Job drawing, mm, ordinate dimensions from the low corner. One solid piece. A direction names the side the tool comes from. Round coordinates to 2 decimals unless told otherwise and drop trailing zeros. Loops run counter-clockwise (first coordinate to the right, second up) from the corner with the lowest first, then second, coordinate; pieces in that order, holes last.
1) Probe line 1 (Z direction, x = 44.41, y = 1); line 2 (X direction, y = 2.95, z = 3.75); line 3 (Z direction, x = 17.5, y = 3.05). List the from-to ranges inside material, lowest first.
2) Band-saw the part on D-D, the plane x = 17.5. Write the cut outline in (y, z).
3) Band-saw the part on A-A, the plane z = 4. Write the cut outline in (x, y), then the cut area to 3 significant figures.
4) Drop flat-ended pins along their axis: P1, Ø1.5, axis at y = 3.5, z = 3, coming from the +X side; P2, Ø3, axis at x = 44.41, z = 4, coming from the +Y side. Give the stop position or say it passes through.
5) Band-saw the part on B-B, the plane x = 4. Write the cut outline in (y, z), then the cut area to 3 significant figures.
6) 3-axis set-ups, long thin cutter, end or side, ignore diameter. For the marked faces 1, 2 and 3: which of +Z, -Z, +X, -X, +Y, -Y reach the whole face in a straight line?
7) Mould opens along X. For the marked faces 4, 5 and 6 say: +X half, -X half, draft (parallel to the pull), parting line (faces both ways), or undercut.
8) Band-saw the part on C-C, the plane y = 1.65. Write the cut outline in (x, z).
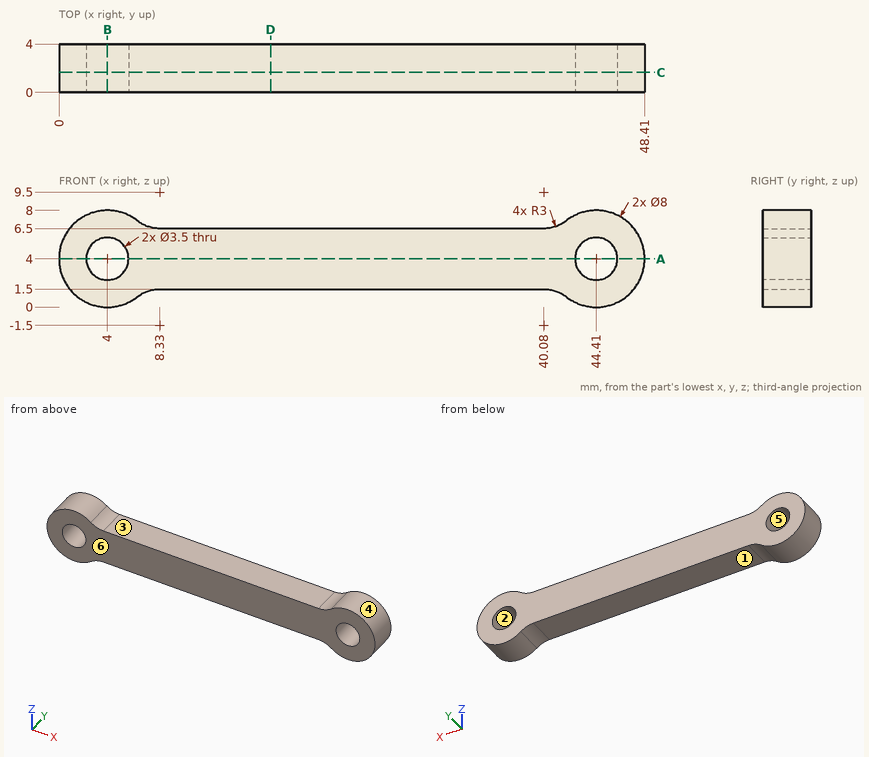
Reported:
1. line 1: z = 0 to 2.25, 5.75 to 8
1. line 2: x = 0.01 to 2.27, 5.73 to 42.68, 46.14 to 48.4
1. line 3: z = 1.5 to 6.5
2. outline: (0, 1.5) - (4, 1.5) - (4, 6.5) - (0, 6.5) - close
3. outline: (0, 0) - (2.25, 0) - (2.25, 4) - (0, 4) - close; (5.75, 0) - (42.66, 0) - (42.66, 4) - (5.75, 4) - close; (46.16, 0) - (48.41, 0) - (48.41, 4) - (46.16, 4) - close
3. area: 166 mm2
4. P1: stops at x = 48.4
4. P2: passes through
5. outline: (0, 0) - (4, 0) - (4, 2.25) - (0, 2.25) - close; (0, 5.75) - (4, 5.75) - (4, 8) - (0, 8) - close
5. area: 18.0 mm2
6. face 1: -Z, +Y, -Y
6. face 2: +Y, -Y
6. face 3: +Z, +Y, -Y
7. face 4: undercut
7. face 5: undercut
7. face 6: draft
8. outline: (6.47, 0.86) arc R3 cw to (8.33, 1.5) - (40.08, 1.5) arc R3 cw to (41.94, 0.86) arc R4 ccw (long way) to (41.94, 7.14) arc R3 cw to (40.08, 6.5) - (8.33, 6.5) arc R3 cw to (6.47, 7.14) arc R4 ccw (long way) to start; hole circle Ø3.5 at (4, 4); hole circle Ø3.5 at (44.41, 4)
